from build123d import *

# Parameters (mm, degrees)
BOSS_EXTRUDE1_DEPTH = 45
SKETCH2_W           = 60
SKETCH2_H           = 30
BOSS_EXTRUDE2_DEPTH = 10
CUT_EXTRUDE1_DEPTH  = 79.262379212
SKETCH4_R           = 10
CUT_EXTRUDE2_DEPTH  = 10
BOSS_EXTRUDE3_DEPTH = 10


with BuildPart() as part:
    # Sketch1 → Boss-Extrude1 (new, symmetric)
    with BuildSketch(Plane(origin=(0, 0, 0), x_dir=(0, 0, -1), z_dir=(1, 0, 0))):
        Polygon((-14.659090909, 0), (15.340909091, 0), (15.340909091, -10), (25.340909091, -10), (25.340909091, 10), (-24.659090909, 10), (-24.659090909, -10), (-14.659090909, -10), align=None)
    extrude(amount=BOSS_EXTRUDE1_DEPTH, both=True)

    # Sketch2 → Boss-Extrude2 (add)
    with BuildSketch(Plane.XY.offset(24.659090909)):
        with Locations((0, 25)):
            Rectangle(SKETCH2_W, SKETCH2_H)
    extrude(amount=-BOSS_EXTRUDE2_DEPTH)

    # Sketch3 → Cut-Extrude1 (cut, through all)
    with BuildSketch(Plane.XY.offset(24.659090909)):
        with BuildLine():
            Line((-10, 23.834240346), (-10, 40))
            Line((-10, 40), (10, 40))
            Line((10, 40), (10, 23.834240346))
            ThreePointArc((10, 23.834240346), (0, 13.834240346), (-10, 23.834240346))
        make_face()
    extrude(amount=-CUT_EXTRUDE1_DEPTH, mode=Mode.SUBTRACT)

    # Sketch4 → Cut-Extrude2 (cut)
    with BuildSketch(Plane(origin=(0, 10, 0), x_dir=(1, 0, 0), z_dir=(0, 1, 0))):
        with Locations(Location((0, 5.340909091, 0), (0, 0, 270))):
            Circle(SKETCH4_R)
    extrude(amount=-CUT_EXTRUDE2_DEPTH, mode=Mode.SUBTRACT)

    # Sketch5 → Boss-Extrude3 (add)
    with BuildSketch(Plane(origin=(30, 0, 0), x_dir=(0, 0, -1), z_dir=(1, 0, 0))):
        Polygon((-14.659090909, 10), (25.340909091, 10), (25.340909091, 20), (-4.659090909, 40), (-14.659090909, 40), align=None)
    extrude(amount=-BOSS_EXTRUDE3_DEPTH)

    # Mirror1: part across plane


with BuildPart() as part_1:
    add(part.part)
    add(part.part.mirror(Plane(origin=(0, 0, 0), x_dir=(0, 0, 1), z_dir=(1, 0, 0))))


solid = part_1.part
Geometry: final body of the model. Coordinates: model frame, mm. A direction names the side the tool comes from. Give positions to 0.01 mm unless a question says otherwise; leave off trailing zeros. Write each loop counter-clockwise with the first axis right and the second up, starting at its lowest first coordinate (ties: lowest second). Pieces come first, ordered by that corner, then holes. Notation, with made-up numbers: (41.5, 30) - (85.5, 30) arc R21 cw to (85.5, 53) - close; hole circle Ø2 at (63.5, 32.5). An arc over 180 degrees is marked (long way). Return JSON: item names as keys, results as strings. Group by question number.
1) Section A-A on y = -6. Return the cut outline in (x, z), plus the area to 3 significant figures.
2) Section C-C on z = 8.5. Return the cut outline in (x, y), plus the area to 3 significant figures.
3) Section B-B on x = -22.5. Return the cut outline in (y, z).
4) First-contact query: P1, Ø9, axis at x = 2.5, y = 18.5, coming from the -Z side; P2, Ø12, axis at x = 0, z = -5.34, coming from the +Y side; P3, Ø2, axis at y = 24.5, z = -12, coming from the -X side; P4, Ø1.5, axis at x = -7.5, z = -11.5, coming from the +Y side. Flat tips, straight axial feed; report the tip coordinate or a pass-through.
5) Mould query, pull axis X, two halves, no side actions, for faces 1 (the flat face through (38, 10, -1)), 2 (the cylindrical face through (0.22, 13.837, 19.729)), 3 (the flat face through (-45, 2, 0)). Classes: released by +X, released by -X, zero draft, split by the parting line, or undercut.
6) Line query: line 1 (X direction, y = 28, z = 8); line 2 (Z direction, x = 0, y = 6.5); line 3 (Z direction, x = 20.5, y = -6.5). Output: solid intervals per line, ascending.
7) Section D-D on y = 5.5. Return the cut outline in (x, z).
8) Set-up query: faces 4 (the flat face through (1, 0, 7)), 5 (the flat face through (-1, 1, -25.341)), 6 (the flat face through (-30, 22, 6)), 7 (the flat face through (5, 10, -15)), 8 (the flat face through (10, 32, 20)). Return all of +Z, -Z, +X, -X, +Y, -Y with unobstructed straight access to the full face (end or side cutting, diameter ignored); none if empty.
Filled in:
{
 "1": {"outline": "(-45, -25.34) - (45, -25.34) - (45, -15.34) - (-45, -15.34) - close; (-45, 14.66) - (45, 14.66) - (45, 24.66) - (-45, 24.66) - close", "area": "1,800 mm^2"},
 "2": {"outline": "(-45, 0) - (45, 0) - (45, 10) - (30, 10) - (30, 40) - (20, 40) - (20, 10) - (-20, 10) - (-20, 40) - (-30, 40) - (-30, 10) - (-45, 10) - close", "area": "1,500 mm^2"},
 "3": {"outline": "(-10, -25.34) - (20, -25.34) - (40, 4.66) - (40, 24.66) - (-10, 24.66) - (-10, 14.66) - (0, 14.66) - (0, -15.34) - (-10, -15.34) - close"},
 "4": {"P1": "stops at z = 14.66", "P2": "passes through", "P3": "stops at x = -30", "P4": "stops at y = 10"},
 "5": {"face 1": "zero draft", "face 2": "undercut", "face 3": "released by -X"},
 "6": {"line 1": "x = -30 to -20, 20 to 30", "line 2": "z = -25.34 to -15.34, 4.66 to 24.66", "line 3": "z = -25.34 to -15.34, 14.66 to 24.66"},
 "7": {"outline": "(-45, -25.34) - (45, -25.34) - (45, 24.66) - (-45, 24.66) - close; hole circle Ø20 at (0, -5.34)"},
 "8": {"face 4": "+X, -X, -Y", "face 5": "-Z, +X, -X, +Y, -Y", "face 6": "+Z, -Z, -X, +Y", "face 7": "-Z, +Y", "face 8": "+Z, -Z, +Y"}
}
